from build123d import *

# Parameters (mm, degrees)
BOSS_EXTRUDE1_DEPTH = 127
CUT_EXTRUDE1_DEPTH  = 10.525


with BuildPart() as part:
    # Sketch1 → Boss-Extrude1 (new body, symmetric)
    with BuildSketch(Plane.XY):
        Polygon((-3.571875, 15.875), (-4.7625, 15.875), (-4.7625, 0), (4.7625, 0), (4.7625, 15.875), (3.571875, 15.875), (3.571875, 1.190625), (-3.571875, 1.190625), align=None)
    extrude(amount=BOSS_EXTRUDE1_DEPTH, both=True)

    # Sketch3 → Cut-Extrude1 (cut, through all)
    with BuildSketch(Plane.ZY.offset(4.7625)):
        Polygon((127, 0), (117.610335596, 14.084496606), (106.170739416, 31.243890876), (157.683078153, 12.341977689), align=None)
    extrude(amount=-CUT_EXTRUDE1_DEPTH, mode=Mode.SUBTRACT)


solid = part.part
The listing builds one solid part. Answer for the finished solid, in the listing's coordinates (mm). A direction names the side the tool comes from. Round coordinates to 2 decimals unless told otherwise and drop trailing zeros. Order: outer loops, then holes, each group sorted by start corner. A loop starts at its lowest first (then second) coordinate and runs counter-clockwise, first axis right, second up. Notation, with made-up numbers: (18, -8.5) - (27, -8.5) arc R20 cw to (27, 18.5) - close; hole circle Ø9 at (10.25, 39.5). An arc over 180 degrees is marked (long way). Write item = value, one per line. Start each with the question number.
1) Section C-C, the plane x = -1.5 is taken. Write down the section's boundary in (y, z), plus the area to 3 significant figures.
2) Section A-A, the plane y = 6 is taken. Write down the section's boundary in (x, z).
3) Given pin 1 (3.5 mm diameter, centred on x = 0.5, z = 39.5, fed in from +Y), flat-ended and moving along its own axis, determine where the tip first touches the part or whether it passes through.
4) For a pull along X with two mould halves and no side action, classify faces 3 (the flat face through (-3.572, 8, 1)), 4 (the flat face through (-4.762, 8, 2)), 5 (the flat face through (4.762, 8, 2)) as released by +X, released by -X, zero draft, split by the parting line, or undercut.
5) For faces 1 (the flat face through (-4, 6, -127)), 2 (the flat face through (3.572, 9, 1)), determine the directions among +Z, -Z, +X, -X, +Y, -Y from which every point of the face is accessible in a straight line to the end or side of a thin tool.
6) Straight lines are drawn through the part: L1, parallel to X at y = 10, z = 96.5; L2, parallel to Y at x = -0.25, z = -27.5; L3, parallel to Z at x = -4, y = 8.5. For each, find the intervals that lie inside material, in ascending order.
7) Section B-B, the plane z = -68.5 is taken. Write down the section's boundary in (x, y) (1 decimal), plus the area to 3 significant figures.
Results list:
q1.outline = (0, -127) - (1.19, -127) - (1.19, 126.21) - (0, 127) - close
q1.area = 302 mm^2
q2.outline = (-4.76, -127) - (-3.57, -127) - (-3.57, 123) - (-4.76, 123) - close; (3.57, -127) - (4.76, -127) - (4.76, 123) - (3.57, 123) - close
q3.pin_1 = 1.19
q4.face_3 = undercut
q4.face_4 = released by -X
q4.face_5 = released by +X
q5.face_1 = -Z, +X, -X, +Y, -Y
q5.face_2 = +Z, -Z, +Y
q6.L1 = -4.76 to -3.57, 3.57 to 4.76
q6.L2 = 0 to 1.19
q6.L3 = -127 to 121.33
q7.outline = (-4.8, 0) - (4.8, 0) - (4.8, 15.9) - (3.6, 15.9) - (3.6, 1.2) - (-3.6, 1.2) - (-3.6, 15.9) - (-4.8, 15.9) - close
q7.area = 46.3 mm^2
